CAD build for the part. Positions are in the model's coordinates, mm. Face numbers are marked on the shaded views. A direction names the side the tool comes from. Coordinates: 2 decimals unless noted, no trailing zeros. Loops run counter-clockwise (first coordinate to the right, second up) from the corner with the lowest first, then second, coordinate; pieces in that order, holes last. Notation, with made-up numbers: (24, -12.5) - (60, -12.5) arc R4 ccw to (60, -5.5) - close; hole circle Ø10 at (87, 37). An arc over 180 degrees is marked (long way). Put each result on its own line as item: value.
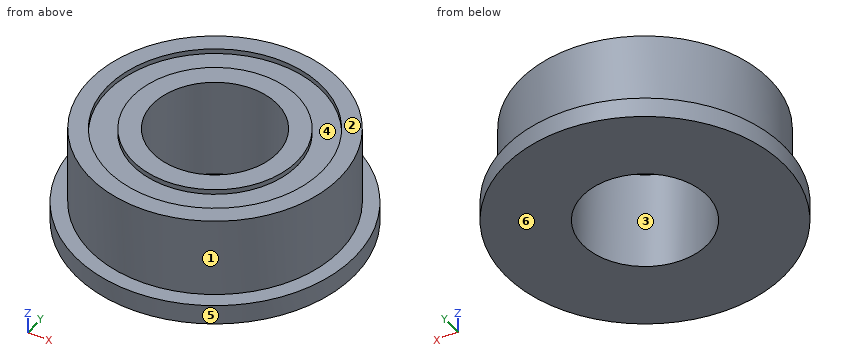
```python
from build123d import *

# Parameters (mm, degrees)
SKETCH1_R        = 5.6
SKETCH1_R_2      = 3.3
FLANGE_DEPTH     = 0.8
SKETCH2_R        = 5
SKETCH2_R_2      = 4.3
OUTER_RING_DEPTH = 3.2
SKETCH3_R        = 3.3
SKETCH3_R_2      = 2.5
INNER_RING_DEPTH = 4
SKETCH4_R        = 4.3
SKETCH4_R_2      = 3.3
SHIELDS_DEPTH    = 2.8


with BuildPart() as part:
    # Sketch1 → Flange (new body)
    with BuildSketch(Plane.XY):
        Circle(SKETCH1_R)
        Circle(SKETCH1_R_2, mode=Mode.SUBTRACT)
    extrude(amount=FLANGE_DEPTH)

    # Sketch2 → Outer_ring (add)
    with BuildSketch(Plane.XY.offset(0.8)):
        Circle(SKETCH2_R)
        Circle(SKETCH2_R_2, mode=Mode.SUBTRACT)
    extrude(amount=OUTER_RING_DEPTH)

    # Sketch3 → Inner_ring (add)
    with BuildSketch(Plane.XY):
        Circle(SKETCH3_R)
        Circle(SKETCH3_R_2, mode=Mode.SUBTRACT)
    extrude(amount=INNER_RING_DEPTH)

    # Sketch4 → Shields (add)
    with BuildSketch(Plane.XY.offset(1)):
        Circle(SKETCH4_R)
        Circle(SKETCH4_R_2, mode=Mode.SUBTRACT)
    extrude(amount=SHIELDS_DEPTH)


solid = part.part
```
Q1. Slice it at A-A, the plane x = 0. Give the cut face in (y, z), then the cut area to 3 significant figures.
Determined:
outline: (-5.6, 0) - (-2.5, 0) - (-2.5, 4) - (-3.3, 4) - (-3.3, 3.8) - (-4.3, 3.8) - (-4.3, 4) - (-5, 4) - (-5, 0.8) - (-5.6, 0.8) - close; (2.5, 0) - (5.6, 0) - (5.6, 0.8) - (5, 0.8) - (5, 4) - (4.3, 4) - (4.3, 3.8) - (3.3, 3.8) - (3.3, 4) - (2.5, 4) - close; hole (-4.3, 0.8) - (-3.3, 0.8) - (-3.3, 1) - (-4.3, 1) - close; hole (3.3, 0.8) - (4.3, 0.8) - (4.3, 1) - (3.3, 1) - close
area: 20.2 mm2
Q2. Tool access for the marked faces 1 and 2: list every direction of +Z, -Z, +X, -X, +Y, -Y with a clear straight run to the whole face (end or side of a thin tool).
Determined:
face 1: +Z
face 2: +Z, +X, -X, +Y, -Y
Q3. Pin check, flat tip, straight feed: pin 1 Ø1.5 at (x, z) = (4, 1) entering from -Y. Stop position of the tip, or through.
Determined:
pin 1: y = -4.54
Q4. Slice it at C-C, the plane y = 3.5. Give the cut face in (x, z), then the cut area to 3 significant figures.
Determined:
outline: (-4.37, 0) - (4.37, 0) - (4.37, 0.8) - (3.57, 0.8) - (3.57, 4) - (2.5, 4) - (2.5, 3.8) - (-2.5, 3.8) - (-2.5, 4) - (-3.57, 4) - (-3.57, 0.8) - (-4.37, 0.8) - close; hole (-2.5, 0.8) - (2.5, 0.8) - (2.5, 1) - (-2.5, 1) - close
area: 27.8 mm2
Q5. Mould opens along Y. For the marked faces 3, 4, 5 and 6 say: +Y half, -Y half, draft (parallel to the pull), parting line (faces both ways), or undercut.
Determined:
face 3: undercut
face 4: undercut
face 5: parting line
face 6: draft
Q6. Slice it at D-D, the plane x = 3.75. Give the cut face in (y, z), then the cut area to 3 significant figures.
Determined:
outline: (-4.16, 0) - (4.16, 0) - (4.16, 0.8) - (3.31, 0.8) - (3.31, 4) - (2.1, 4) - (2.1, 3.8) - (-2.1, 3.8) - (-2.1, 4) - (-3.31, 4) - (-3.31, 0.8) - (-4.16, 0.8) - close; hole (-2.1, 0.8) - (2.1, 0.8) - (2.1, 1) - (-2.1, 1) - close
area: 26.1 mm2
Q7. Wall check: L1, parallel to Y at x = 0, z = 3.9; L2, parallel to Z at x = 0.75, y = -3.75; L3, parallel to Y at x = 0, z = 1.7. Give the ranges that are in metal, low to high. Write a range as from..to.
Determined:
L1: -5..-4.3, -3.3..-2.5, 2.5..3.3, 4.3..5
L2: 0..0.8, 1..3.8
L3: -5..-2.5, 2.5..5
